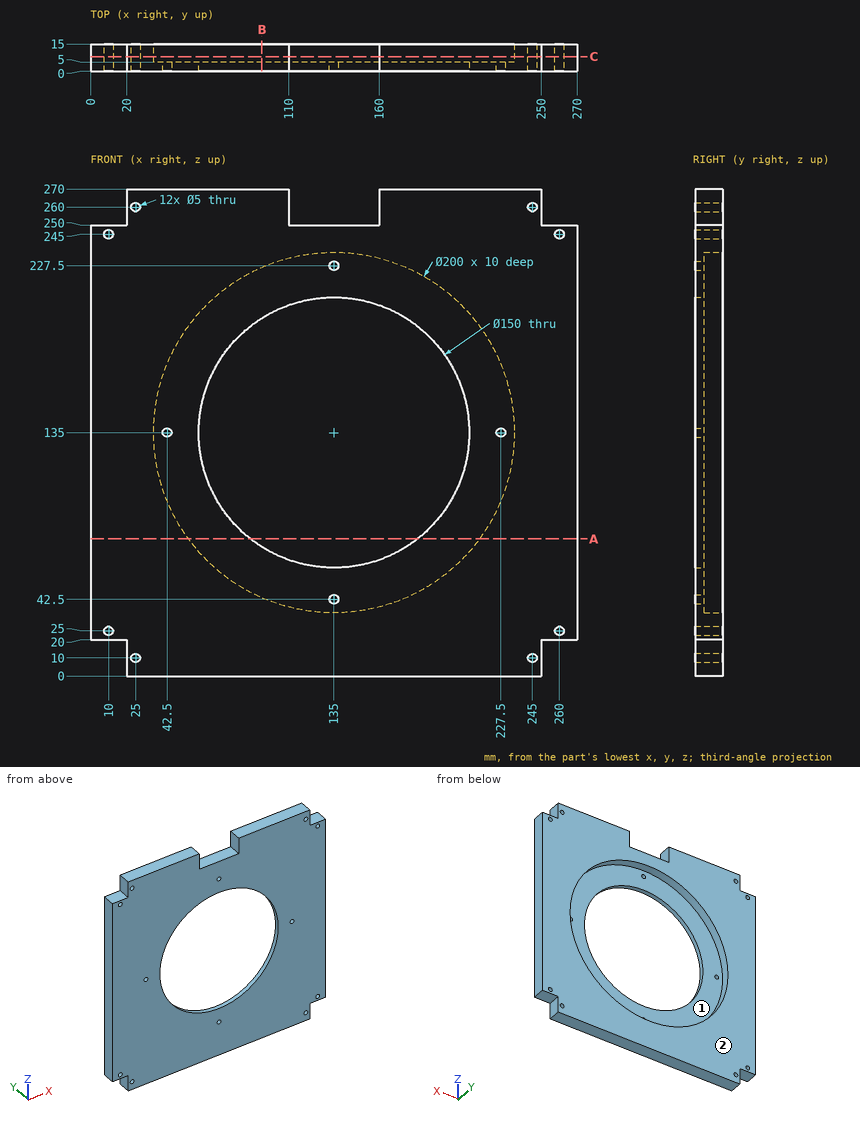
Source: three-view drawing plus pictorial views. Frame: mm from the lowest corner of the part. Coordinates: 2 decimals unless noted, no trailing zeros. Loops run counter-clockwise (first coordinate to the right, second up) from the corner with the lowest first, then second, coordinate; pieces in that order, holes last. Notation, with made-up numbers: (-6.75, 77.25) - (12.25, 77.25) arc R27 cw to (12.25, 107.25) - close; hole circle Ø7 at (79, -24.75). An arc over 180 degrees is marked (long way). One line per item, written item: value. Start each with the question number.
1. Mould query, pull axis X, two halves, no side actions, for the marked faces 1 and 2. Classes: pulls with the +X half, pulls with the -X half, needs draft (parallel to the pull), parting line crosses it, or undercut.
2. Section B-B (x = 95). Return the cut outline in (y, z).
3. Ray query, L1, parallel to Z at x = 135, y = 1.4; L2, parallel to Z at x = 10, y = 7; L3, parallel to X at y = 1.1, z = 135. Return the intervals inside material, ascending.
4. Section A-A (z = 76). Return the cut outline in (x, y).
5. Contact query for flat-ended pins moving along their axis: P1, Ø4.5, axis at y = 4, z = 257.5, coming from the -X side; P2, Ø7.5, axis at y = 6, z = 260, coming from the +X side; P3, Ø6.5, axis at x = 42.5, z = 135, coming from the +Y side. Output: stop coordinate, or through.
6. Section C-C (y = 8). State how many separate pieces and enclosed holes the cut face has, and give its area (3 significant figures).
Verdict:
1. face 1: undercut
1. face 2: needs draft
2. outline: (0, 0) - (15, 0) - (15, 43.35) - (5, 43.35) - (5, 71.56) - (0, 71.56) - close; (0, 198.44) - (5, 198.44) - (5, 226.65) - (15, 226.65) - (15, 270) - (0, 270) - close
3. L1: z = 0 to 40, 45 to 60, 210 to 225, 230 to 250
3. L2: z = 20 to 22.5, 27.5 to 242.5, 247.5 to 250
3. L3: x = 0 to 40, 45 to 60, 210 to 225, 230 to 270
4. outline: (0, 0) - (88.7, 0) - (88.7, 5) - (54.26, 5) - (54.26, 15) - (0, 15) - close; (181.3, 0) - (270, 0) - (270, 15) - (215.74, 15) - (215.74, 5) - (181.3, 5) - close
5. P1: stops at x = 20
5. P2: stops at x = 250
5. P3: stops at y = 5
6. separate pieces: 1
6. enclosed holes: 9
6. area: 38,700 mm2
